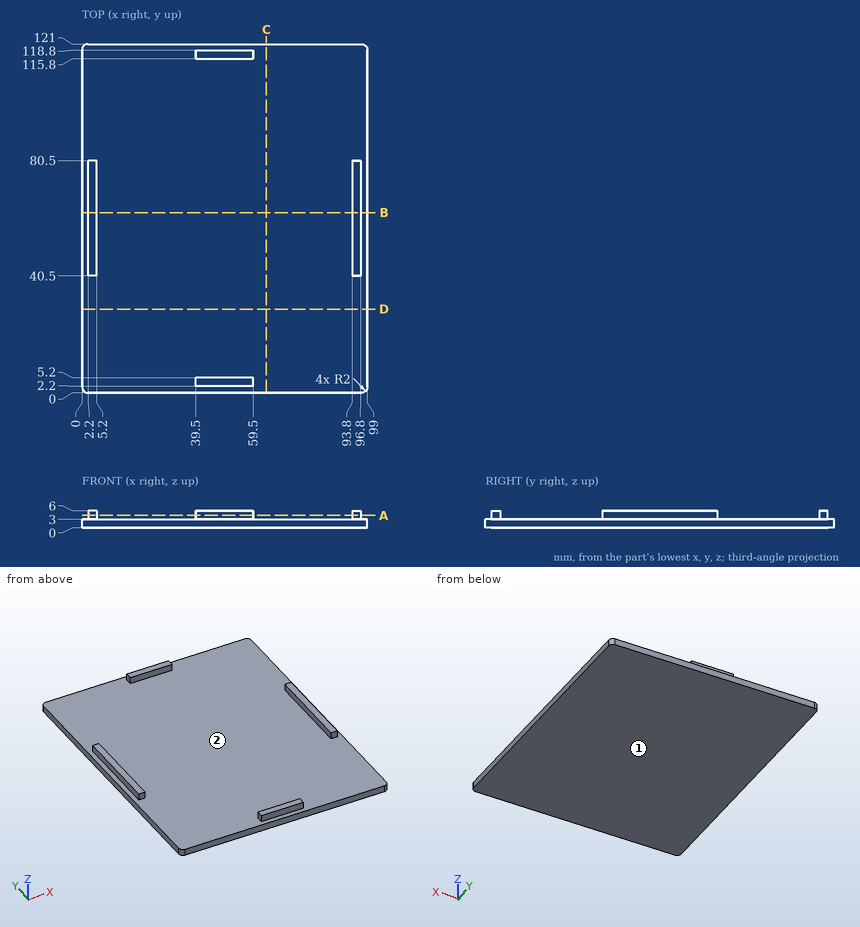
Can you work these out from the drawing? Everything is in mm from the part's minimum corner. Coordinates: 2 decimals unless noted, no trailing zeros. Loops run counter-clockwise (first coordinate to the right, second up) from the corner with the lowest first, then second, coordinate; pieces in that order, holes last. Notation, with made-up numbers: M -24,30 L 9,30 A13 ccw 9,49 Z; hole C 42.5,50.5 d5. An arc over 180 degrees is marked long. One line per item, written item: value.
1. Will these pins go through, and if not, where does the flat tip stop? pin 1 Ø1.5 at (x, z) = (51, 4.5) entering from +Y; pin 2 Ø1.5 at (y, z) = (4, 4) entering from -X; pin 3 Ø0.9 at (x, z) = (95, 5) entering from -Y.
Geometry says:
pin 1: stops at y = 118.8
pin 2: stops at x = 39.5
pin 3: stops at y = 40.5
2. Imagine slicing it at D-D (y = 29). List the corners of the cut face in (x, z) for me.
Geometry says:
outline: M 0,0 L 99,0 L 99,3 L 0,3 Z
3. Imagine slicing it at C-C (x = 64). List the corners of the cut face in (y, z) for me.
Geometry says:
outline: M 0,0 L 121,0 L 121,3 L 0,3 Z
4. Please list where these lines run through material, in increasing order: probe 1 along Y at (x, z) = (43.5, 5.35); probe 2 along Z at (x, y) = (52.5, 52); probe 3 along X at (y, z) = (72.5, 5.15).
Geometry says:
probe 1: y = 2.2 to 5.2, 115.8 to 118.8
probe 2: z = 0 to 3
probe 3: x = 2.2 to 5.2, 93.8 to 96.8
5. Thinking about a two-plate mould opening in X: for the marked faces 1 and 2, which applies, +X half, -X half, draft (parallel to the pull), parting line (faces both ways), or undercut?
Geometry says:
face 1: draft
face 2: undercut
6. Imagine slicing it at B-B (y = 62.5). List the corners of the cut face in (x, z) for me.
Geometry says:
outline: M 0,0 L 99,0 L 99,3 L 96.8,3 L 96.8,6 L 93.8,6 L 93.8,3 L 5.2,3 L 5.2,6 L 2.2,6 L 2.2,3 L 0,3 Z
7. Imagine slicing it at A-A (z = 4.35). List the corners of the cut face in (x, y) for me, and give its area (3 significant figures).
Geometry says:
outline: M 2.2,40.5 L 5.2,40.5 L 5.2,80.5 L 2.2,80.5 Z; M 39.5,2.2 L 59.5,2.2 L 59.5,5.2 L 39.5,5.2 Z; M 39.5,115.8 L 59.5,115.8 L 59.5,118.8 L 39.5,118.8 Z; M 93.8,40.5 L 96.8,40.5 L 96.8,80.5 L 93.8,80.5 Z
area: 360 mm2
